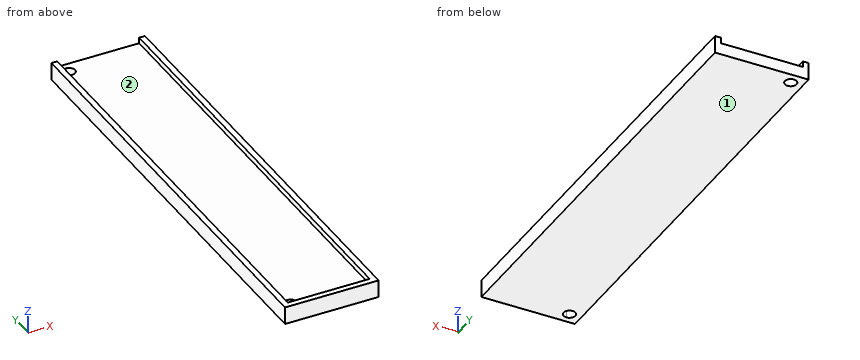
```python
from build123d import *

# Parameters (mm, degrees)
F0_W     = 3.175
F0_H     = 3.175
F0_H_2   = 234.95
F1_DEPTH = 9.525
F2_DEPTH = 6.35
F3_DEPTH = 6.35


with BuildPart() as f1:
    # F0 (on Top) → F1 (new body)
    with BuildSketch(Plane.XY):
        with Locations((-45.285827, 169.703753)):
            Rectangle(F0_W, F0_H)
        Polygon((-43.698327, 168.116253), (-46.873327, 168.116253), (-46.873327, 158.591253), (-46.873327, -57.308747), (-46.873327, -66.833747), (-43.698327, -66.833747), (-43.698327, -63.658747), (-43.698327, 164.941253), align=None)
        with Locations((2.339173, 169.703753)):
            Rectangle(F0_W, F0_H)
        with Locations((2.339173, 50.641253)):
            Rectangle(F0_W, F0_H_2)
        with Locations((-45.285827, -68.421247)):
            Rectangle(F0_W, F0_H)
        Polygon((0.751673, -70.008747), (0.751673, -66.833747), (-40.523327, -66.833747), (-43.698327, -66.833747), (-43.698327, -70.008747), (-34.173327, -70.008747), align=None)
        with Locations((2.339173, -68.421247)):
            Rectangle(F0_W, F0_H)
    extrude(amount=F1_DEPTH)

    # F0 (on Top) → F2 (join)
    with BuildSketch(Plane.XY):
        with BuildLine():
            ThreePointArc((-37.348327, 164.941253), (-40.523327, 161.766253), (-43.698327, 164.941253))
            Line((-43.698327, 164.941253), (-43.698327, -63.658747))
            ThreePointArc((-43.698327, -63.658747), (-40.523327, -60.483747), (-37.348327, -63.658747))
            ThreePointArc((-37.348327, -63.658747), (-38.278263, -65.903811), (-40.523327, -66.833747))
            Line((-40.523327, -66.833747), (0.751673, -66.833747))
            Line((0.751673, -66.833747), (0.751673, 168.116253))
            Line((0.751673, 168.116253), (-40.523327, 168.116253))
            ThreePointArc((-40.523327, 168.116253), (-38.278263, 167.186317), (-37.348327, 164.941253))
        make_face()
        Polygon((-34.173327, 171.291253), (-43.698327, 171.291253), (-43.698327, 168.116253), (-40.523327, 168.116253), (0.751673, 168.116253), (0.751673, 171.291253), align=None)
    extrude(amount=F2_DEPTH)

    # F0 (on Top) → F3 (join)
    with BuildSketch(Plane.XY):
        with BuildLine():
            Line((-40.523327, 168.116253), (-43.698327, 168.116253))
            Line((-43.698327, 168.116253), (-43.698327, 164.941253))
            ThreePointArc((-43.698327, 164.941253), (-42.768391, 167.186317), (-40.523327, 168.116253))
        make_face()
        with BuildLine():
            ThreePointArc((-40.523327, -66.833747), (-42.768391, -65.903811), (-43.698327, -63.658747))
            Line((-43.698327, -63.658747), (-43.698327, -66.833747))
            Line((-43.698327, -66.833747), (-40.523327, -66.833747))
        make_face()
    extrude(amount=F3_DEPTH)


solid = f1.part
```
Geometry check sheet. Reference: the model listing, model coordinates, mm. Face numbers are marked on the shaded views. Coordinates: 2 decimals unless noted, no trailing zeros. Write each loop counter-clockwise with the first axis right and the second up, starting at its lowest first coordinate (ties: lowest second). Pieces come first, ordered by that corner, then holes. Notation, with made-up numbers: M 80,-14.75 L 124,-14.75 A16 ccw 124,-4.75 Z; hole C 8,74.25 d10. An arc over 180 degrees is marked long. One line per item, written item: value. Start each with the question number.
(1) Sectioned sample at A-A, the plane y = 156. Enter the section's corners in (x, z) (3 decimals).
(2) Scan lines: line 1 along X through (y, z) = (149.5, 7.75); line 2 along Y through (x, z) = (-1, 7); line 3 along Z through (x, y) = (-6, 126). Record each from-to range of solid material in increasing order. Write a range as [from, to].
(3) Sectioned sample at B-B, the plane x = -21. Enter the section's corners in (y, z) (3 decimals), and give its area (3 significant figures).
(4) Depth check by flat-ended pin: pin 1 (3.5 mm diameter, centred on x = -29.5, z = 7.5, fed in from +Y); pin 2 (1 mm diameter, centred on x = -41.5, y = -65, fed in from +Z); pin 3 (22 mm diameter, centred on x = -15.5, y = 77.5, fed in from +Z). Enter the tip coordinate at first touch or a pass-through.
(5) Release check for a two-part mould opening along X. For the marked faces 1 and 2 record: released by +X, released by -X, zero draft, split by the parting line, or undercut.
Filled sheet:
1. outline: M -46.873,0 L 3.927,0 L 3.927,9.525 L 0.752,9.525 L 0.752,6.35 L -43.698,6.35 L -43.698,9.525 L -46.873,9.525 Z
2. line 1: [-46.87, -43.7], [0.75, 3.93]
2. line 2: [-70.01, -66.83]
2. line 3: [0, 6.35]
3. outline: M -70.009,0 L 171.291,0 L 171.291,6.35 L -66.834,6.35 L -66.834,9.525 L -70.009,9.525 Z
3. area: 1,540 mm²
4. pin 1: y = 171.29
4. pin 2: through
4. pin 3: z = 6.35
5. face 1: zero draft
5. face 2: undercut
